Verification items for the finished model (mm, model axes). Coordinates: 2 decimals unless noted, no trailing zeros. Order: outer loops, then holes, each group sorted by start corner. A loop starts at its lowest first (then second) coordinate and runs counter-clockwise, first axis right, second up. Notation, with made-up numbers: M 7,57 L 56,57 A29 ccw 56,85 Z; hole C 35.25,-17.75 d8. An arc over 180 degrees is marked long. Write item = value, one per line.
```python
from build123d import *

# Parameters (mm, degrees)
BOSS_EXTRUDE1_DEPTH = 5
SKETCH2_R           = 4
CUT_EXTRUDE1_DEPTH  = 5
CUT_EXTRUDE4_DEPTH  = 35


with BuildPart() as part:
    # Sketch1 → Boss-Extrude1 (new body)
    with BuildSketch(Plane.XY):
        with BuildLine():
            Line((115.454232837, -90), (-115.454232837, -90))
            ThreePointArc((-115.454232837, -90), (-121.637702261, -87.85905248), (-125.173474979, -82.352941176))
            ThreePointArc((-125.173474979, -82.352941176), (-135, 0), (-125.173474979, 82.352941176))
            ThreePointArc((-125.173474979, 82.352941176), (-121.637702261, 87.85905248), (-115.454232837, 90))
            Line((-115.454232837, 90), (115.454232837, 90))
            ThreePointArc((115.454232837, 90), (121.637702261, 87.85905248), (125.173474979, 82.352941176))
            ThreePointArc((125.173474979, 82.352941176), (135, 0), (125.173474979, -82.352941176))
            ThreePointArc((125.173474979, -82.352941176), (121.637702261, -87.85905248), (115.454232837, -90))
        make_face()
    extrude(amount=BOSS_EXTRUDE1_DEPTH)

    # Sketch2 → Cut-Extrude1 (cut)
    with BuildSketch(Plane.XY.offset(5)):
        with Locations((0, 22.8)):
            Circle(SKETCH2_R)
        with Locations((19.745379206, -11.4)):
            Circle(SKETCH2_R)
        with Locations((-19.745379206, -11.4)):
            Circle(SKETCH2_R)
    extrude(amount=-CUT_EXTRUDE1_DEPTH, mode=Mode.SUBTRACT)

    # Sketch4 → Cut-Extrude4 (cut)
    with BuildSketch(Plane.XY.offset(5)):
        with BuildLine():
            Line((92.589613382, 7.756373084), (108.233016215, 1.740021021))
            ThreePointArc((108.233016215, 1.740021021), (120.339926562, -8.155270139), (124.200171868, -23.307582551))
            ThreePointArc((124.200171868, -23.307582551), (121.709079907, -47.191053261), (117.538445446, -70.839129726))
            ThreePointArc((117.538445446, -70.839129726), (113.463443203, -76.968226609), (106.297665816, -78.648436814))
            Line((106.297665816, -78.648436814), (87.539762883, -75.879659935))
            ThreePointArc((87.539762883, -75.879659935), (81.430245342, -72.521282016), (79, -65.986849032))
            Line((79, -65.986849032), (79, -1.577151211))
            ThreePointArc((79, -1.577151211), (83.338557331, 6.665910532), (92.589613382, 7.756373084))
        make_face()
        with BuildLine():
            ThreePointArc((-92.589613382, 7.756373084), (-83.338557331, 6.665910532), (-79, -1.577151211))
            Line((-79, -1.577151211), (-79, -65.986849032))
            ThreePointArc((-79, -65.986849032), (-81.430245342, -72.521282016), (-87.539762883, -75.879659935))
            Line((-87.539762883, -75.879659935), (-106.297665816, -78.648436814))
            ThreePointArc((-106.297665816, -78.648436814), (-113.463443203, -76.968226609), (-117.538445446, -70.839129726))
            ThreePointArc((-117.538445446, -70.839129726), (-121.709079907, -47.191053261), (-124.200171868, -23.307582551))
            ThreePointArc((-124.200171868, -23.307582551), (-120.339926562, -8.155270139), (-108.233016215, 1.740021021))
            Line((-108.233016215, 1.740021021), (-92.589613382, 7.756373084))
        make_face()
        with BuildLine():
            add(Edge.make_bspline(
                [(-107.1656403, 63.712244747), (-105.421734613, 63.094579339), (-103.733740594, 62.553921113), (-100.607161167, 61.582975733), (-99.159247663, 61.147865372), (-96.410321129, 60.288497128), (-95.109448347, 59.864130878), (-92.675824035, 58.977926734), (-91.543513421, 58.51617249), (-89.457956468, 57.516788843), (-88.505180062, 56.979898005), (-86.763629608, 55.791229907), (-85.974064887, 55.140456421), (-84.517341855, 53.654449203), (-83.848519279, 52.818369685), (-82.607884183, 50.851859219), (-82.036322501, 49.719874222), (-81.010476423, 47.056406193), (-80.557249512, 45.52494381), (-79.807126347, 41.990071718), (-79.510581534, 39.987228491), (-79.107044911, 35.456158677), (-79, 32.928236614), (-79, 30.112884289)],
                knots=[0.308064858, 0.308064858, 0.308064858, 0.308064858, 0.375, 0.375, 0.4375, 0.4375, 0.5, 0.5, 0.5625, 0.5625, 0.625, 0.625, 0.6875, 0.6875, 0.75, 0.75, 0.8125, 0.8125, 0.875, 0.875, 0.9375, 0.9375, 1, 1, 1, 1], degree=3))
            Line((-79, 30.112884289), (-79, 22.274807415))
            ThreePointArc((-79, 22.274807415), (-80.264551221, 18.95119155), (-83.418568967, 17.308728685))
            Line((-83.418568967, 17.308728685), (-98.190518564, 15.579221284))
            ThreePointArc((-98.190518564, 15.579221284), (-104.024603132, 16.045769918), (-109.236054023, 18.709412158))
            Line((-109.236054023, 18.709412158), (-117.213085535, 25.01430829))
            ThreePointArc((-117.213085535, 25.01430829), (-121.761034531, 31.020418271), (-122.815466707, 38.480000696))
            ThreePointArc((-122.815466707, 38.480000696), (-121.704826963, 47.22138816), (-120.368031746, 55.931058302))
            ThreePointArc((-120.368031746, 55.931058302), (-115.58177318, 62.901067623), (-107.1656403, 63.712244747))
        make_face()
        with BuildLine():
            add(Edge.make_bspline(
                [(107.1656403, 63.712244747), (105.421734613, 63.094579339), (103.733740594, 62.553921113), (100.607161167, 61.582975733), (99.159247663, 61.147865372), (96.410321129, 60.288497128), (95.109448347, 59.864130878), (92.675824035, 58.977926734), (91.543513421, 58.51617249), (89.457956468, 57.516788843), (88.505180062, 56.979898005), (86.763629608, 55.791229907), (85.974064887, 55.140456421), (84.517341855, 53.654449203), (83.848519279, 52.818369685), (82.607884183, 50.851859219), (82.036322501, 49.719874222), (81.010476423, 47.056406193), (80.557249512, 45.52494381), (79.807126347, 41.990071718), (79.510581534, 39.987228491), (79.107044911, 35.456158677), (79, 32.928236614), (79, 30.112884289)],
                knots=[0.308064858, 0.308064858, 0.308064858, 0.308064858, 0.375, 0.375, 0.4375, 0.4375, 0.5, 0.5, 0.5625, 0.5625, 0.625, 0.625, 0.6875, 0.6875, 0.75, 0.75, 0.8125, 0.8125, 0.875, 0.875, 0.9375, 0.9375, 1, 1, 1, 1], degree=3))
            Line((79, 30.112884289), (79, 22.274807415))
            ThreePointArc((79, 22.274807415), (80.264551221, 18.95119155), (83.418568967, 17.308728685))
            Line((83.418568967, 17.308728685), (98.190518564, 15.579221284))
            ThreePointArc((98.190518564, 15.579221284), (104.024603132, 16.045769918), (109.236054023, 18.709412158))
            Line((109.236054023, 18.709412158), (117.213085535, 25.01430829))
            ThreePointArc((117.213085535, 25.01430829), (121.761034531, 31.020418271), (122.815466707, 38.480000696))
            ThreePointArc((122.815466707, 38.480000696), (121.704826963, 47.22138816), (120.368031746, 55.931058302))
            ThreePointArc((120.368031746, 55.931058302), (115.58177318, 62.901067623), (107.1656403, 63.712244747))
        make_face()
    extrude(amount=-CUT_EXTRUDE4_DEPTH, mode=Mode.SUBTRACT)


solid = part.part
```
Item 1: Sectioned sample at C-C, the plane y = -11.4. Enter the section's corners in (x, z).
Report:
outline = M -134.81,0 L -122.09,0 L -122.09,5 L -134.81,5 Z; M -79,0 L -23.75,0 L -23.75,5 L -79,5 Z; M -15.75,0 L 15.75,0 L 15.75,5 L -15.75,5 Z; M 23.75,0 L 79,0 L 79,5 L 23.75,5 Z; M 122.09,0 L 134.81,0 L 134.81,5 L 122.09,5 Z
Item 2: Gauge pin test, flat ends, axial feed: pin 1 (5 mm diameter, centred on x = 0, y = 22.8, fed in from -Z); pin 2 (1 mm diameter, centred on y = -59.5, z = 1.5, fed in from -X); pin 3 (1.5 mm diameter, centred on y = 26.5, z = 3, fed in from -X); pin 4 (3 mm diameter, centred on y = -13, z = 3, fed in from +X). Record the tip position at first contact, or that the pin passes through.
Report:
pin_1 = through
pin_2 = -129.99
pin_3 = -134.05
pin_4 = 134.81
Item 3: Sectioned sample at A-A, the plane x = 0. Enter the section's corners in (y, z), then the cut area to 3 significant figures.
Report:
outline = M -90,0 L 18.8,0 L 18.8,5 L -90,5 Z; M 26.8,0 L 90,0 L 90,5 L 26.8,5 Z
area = 860 mm^2
Item 4: Scan lines: L1, parallel to Y at x = -113.5, z = 3.5; L2, parallel to X at y = -30.5, z = 4.6; L3, parallel to Y at x = 96, z = 3.3. Record each from-to range of solid material in increasing order. Write a range as from..to.
Report:
L1 = -90..-76.94, -1.05..22.08, 63.83..90
L2 = -133.67..-123.63, -79..79, 123.63..133.67
L3 = -90..-77.13, 6.44..15.84, 60.15..90
Item 5: Sectioned sample at D-D, the plane y = 77.5. Enter the section's corners in (x, z), then the cut area to 3 significant figures.
Report:
outline = M -126.31,0 L 126.31,0 L 126.31,5 L -126.31,5 Z
area = 1,260 mm^2
Item 6: Release check for a two-part mould opening along Y. For faces 1 (the flat face through (2, 1, 5)), 2 (the cylindrical face through (135, 1, 2)), 3 (the cylindrical face through (113.55, -76.908, 2.535)) record: pulls with the +Y half, pulls with the -Y half, needs draft (parallel to the pull), parting line crosses it, or undercut.
Report:
face_1 = needs draft
face_2 = parting line crosses it
face_3 = undercut
Item 7: Sectioned sample at B-B, the plane z = 4.2. Give the number of separate pieces and of enclosed holes in the cut face, then the cut area to 3 significant figures.
Report:
separate_pieces = 1
enclosed_holes = 7
area = 36,800 mm^2
